Design review of the part built by this model. Coordinates are the model's own, in mm. A direction names the side the tool comes from. Coordinates: 2 decimals unless noted, no trailing zeros. Loops run counter-clockwise (first coordinate to the right, second up) from the corner with the lowest first, then second, coordinate; pieces in that order, holes last. Notation, with made-up numbers: M 12,57.5 L 27,57.5 A32 cw 27,84.5 Z; hole C 26,4 d11. An arc over 180 degrees is marked long. One line per item, written item: value.
```python
from build123d import *
from build123d.topology import SkipClean

# Parameters (mm, degrees)
SKETCH2_R                                = 10
SKETCH2_R_2                              = 6
SKETCH2_R_3                              = 5
BOSS_EXTRUDE1_DEPTH                      = 2
BOSS_EXTRUDE2_START                      = -3
SKETCH2_3_R                              = 21
SKETCH2_3_R_2                            = 20
SKETCH2_3_R_3                            = 17
SKETCH2_3_R_4                            = 10
SKETCH2_3_R_5                            = 6
SKETCH2_3_R_6                            = 5
BOSS_EXTRUDE2_DEPTH                      = 3
BOSS_EXTRUDE3_START                      = -4
SKETCH2_4_R                              = 6
SKETCH2_4_R_2                            = 5
BOSS_EXTRUDE3_DEPTH                      = 4
SKETCH2_6_R                              = 20
SKETCH2_6_R_2                            = 17
BOSS_EXTRUDE4_DEPTH                      = 14
CBORE_FOR_M12_HEX_HEAD_BOLT1_D           = 3.6
CBORE_FOR_M12_HEX_HEAD_BOLT1_CBORE_D     = 6.7
CBORE_FOR_M12_HEX_HEAD_BOLT1_CBORE_DEPTH = 1.65
CIRPATTERN1_COUNT                        = 3
RIB1_REACH                               = 44.5
SKETCH4_WALL_W                           = 101.866218182
SKETCH4_WALL_H                           = 2
CIRPATTERN2_COUNT                        = 6


with BuildPart() as part:
    # Sketch2 → Boss-Extrude1 (new body)
    # profile 1 of 2: a face of its own
    with BuildSketch(Plane(origin=(0, 0, 0), x_dir=(1, 0, 0), z_dir=(0, 1, 0))):
        with Locations(Location((0, 0, 0), (0, 0, 270))):
            Circle(SKETCH2_R)
        Circle(SKETCH2_R_2, mode=Mode.SUBTRACT)
    # profile 2 of 2: a face of its own
    with BuildSketch(Plane(origin=(0, 0, 0), x_dir=(1, 0, 0), z_dir=(0, 1, 0))):
        Circle(SKETCH2_R_2)
        with Locations(Location((0, 0, 0), (0, 0, 270))):
            Circle(SKETCH2_R_3, mode=Mode.SUBTRACT)
    extrude(amount=BOSS_EXTRUDE1_DEPTH)

    # Sketch2_3 → Boss-Extrude2 (add)
    # profile 1 of 8: a face of its own
    with BuildSketch(Plane(origin=(0, 0, 0), x_dir=(1, 0, 0), z_dir=(0, 1, 0)).offset(BOSS_EXTRUDE2_START)):
        with BuildLine():
            ThreePointArc((-15.163521733, -14.528166046), (-18.186533479, -10.5), (-20.163521733, -5.867912008))
            Line((-20.163521733, -5.867912008), (-24.150635095, -8.169872981))
            ThreePointArc((-24.150635095, -8.169872981), (-25.980762114, -15), (-19.150635095, -16.830127019))
            Line((-19.150635095, -16.830127019), (-15.163521733, -14.528166046))
        make_face()
    # profile 2 of 8: a face of its own
    with BuildSketch(Plane(origin=(0, 0, 0), x_dir=(1, 0, 0), z_dir=(0, 1, 0)).offset(BOSS_EXTRUDE2_START)):
        with BuildLine():
            Line((24.150635095, -8.169872981), (20.163521733, -5.867912008))
            ThreePointArc((20.163521733, -5.867912008), (18.186533479, -10.5), (15.163521733, -14.528166046))
            Line((15.163521733, -14.528166046), (19.150635095, -16.830127019))
            ThreePointArc((19.150635095, -16.830127019), (25.980762114, -15), (24.150635095, -8.169872981))
        make_face()
    # profile 3 of 8: a face of its own
    with BuildSketch(Plane(origin=(0, 0, 0), x_dir=(1, 0, 0), z_dir=(0, 1, 0)).offset(BOSS_EXTRUDE2_START)):
        with BuildLine():
            Line((5, 20.396078054), (5, 25))
            ThreePointArc((5, 25), (0, 30), (-5, 25))
            Line((-5, 25), (-5, 20.396078054))
            ThreePointArc((-5, 20.396078054), (0, 21), (5, 20.396078054))
        make_face()
    # profile 4 of 8: a face of its own
    with BuildSketch(Plane(origin=(0, 0, 0), x_dir=(1, 0, 0), z_dir=(0, 1, 0)).offset(BOSS_EXTRUDE2_START)):
        Circle(SKETCH2_3_R)
        Circle(SKETCH2_3_R_2, mode=Mode.SUBTRACT)
    # profile 5 of 8: a face of its own
    with BuildSketch(Plane(origin=(0, 0, 0), x_dir=(1, 0, 0), z_dir=(0, 1, 0)).offset(BOSS_EXTRUDE2_START)):
        Circle(SKETCH2_3_R_2)
        Circle(SKETCH2_3_R_3, mode=Mode.SUBTRACT)
    # profile 6 of 8: a face of its own
    with BuildSketch(Plane(origin=(0, 0, 0), x_dir=(1, 0, 0), z_dir=(0, 1, 0)).offset(BOSS_EXTRUDE2_START)):
        Circle(SKETCH2_3_R_3)
        with Locations(Location((0, 0, 0), (0, 0, 270))):
            Circle(SKETCH2_3_R_4, mode=Mode.SUBTRACT)
    # profile 7 of 8: a face of its own
    with BuildSketch(Plane(origin=(0, 0, 0), x_dir=(1, 0, 0), z_dir=(0, 1, 0)).offset(BOSS_EXTRUDE2_START)):
        with Locations(Location((0, 0, 0), (0, 0, 270))):
            Circle(SKETCH2_3_R_4)
        Circle(SKETCH2_3_R_5, mode=Mode.SUBTRACT)
    # profile 8 of 8: a face of its own
    with BuildSketch(Plane(origin=(0, 0, 0), x_dir=(1, 0, 0), z_dir=(0, 1, 0)).offset(BOSS_EXTRUDE2_START)):
        Circle(SKETCH2_3_R_5)
        with Locations(Location((0, 0, 0), (0, 0, 270))):
            Circle(SKETCH2_3_R_6, mode=Mode.SUBTRACT)
    extrude(amount=BOSS_EXTRUDE2_DEPTH)

    # Sketch2_4 → Boss-Extrude3 (add)
    with BuildSketch(Plane(origin=(0, 0, 0), x_dir=(1, 0, 0), z_dir=(0, 1, 0)).offset(BOSS_EXTRUDE3_START)):
        with Locations(Location((0, 0, 0), (0, 0, 270))):
            Circle(SKETCH2_4_R)
        with Locations(Location((0, 0, 0), (0, 0, 270))):
            Circle(SKETCH2_4_R_2, mode=Mode.SUBTRACT)
    extrude(amount=BOSS_EXTRUDE3_DEPTH)

    # Sketch2_6 → Boss-Extrude4 (add)
    with BuildSketch(Plane(origin=(0, 0, 0), x_dir=(1, 0, 0), z_dir=(0, 1, 0))):
        with Locations(Location((0, 0, 0), (0, 0, 270))):
            Circle(SKETCH2_6_R)
        with Locations(Location((0, 0, 0), (0, 0, 270))):
            Circle(SKETCH2_6_R_2, mode=Mode.SUBTRACT)
    extrude(amount=-BOSS_EXTRUDE4_DEPTH)

    # CBORE for M12 Hex Head Bolt1 (through all)
    with Locations(Plane(origin=(0, 0, -25), x_dir=(0, 0, 1), z_dir=(0, 1, 0))):
        with Locations((0, 0)):
            cbore_for_m12_hex_head_bolt1 = CounterBoreHole(CBORE_FOR_M12_HEX_HEAD_BOLT1_D / 2, CBORE_FOR_M12_HEX_HEAD_BOLT1_CBORE_D / 2, CBORE_FOR_M12_HEX_HEAD_BOLT1_CBORE_DEPTH)

    # CirPattern1: CBORE for M12 Hex Head Bolt1 ×3 about axis
    cirpattern1_axis = Axis((0, 0, 0), (0, 1, 0))
    for i in range(1, CIRPATTERN1_COUNT):
        add(cbore_for_m12_hex_head_bolt1.rotate(cirpattern1_axis, i * 360 / CIRPATTERN1_COUNT), mode=Mode.SUBTRACT)

    # Sketch4 wall → Rib1 (add, up to next)
    with BuildSketch(Plane(origin=(-11.5, -9, 0), x_dir=(0.739940073396, 0.672672793996, 0), z_dir=(-0.672672793996, 0.739940073396, 0)), mode=Mode.PRIVATE) as rib1_sk1:
        Rectangle(SKETCH4_WALL_W, SKETCH4_WALL_H)
    rib1_tool1 = extrude(rib1_sk1.sketch, amount=RIB1_REACH, mode=Mode.PRIVATE) - part.part
    rib1 = rib1_tool1.solids().sort_by_distance((-11.5, -9, 0))[0]
    add(rib1)

    # CirPattern2: Rib1 ×6 about axis
    with SkipClean():  # the faces are left unmerged after this step: merging them gives an invalid solid
        cirpattern2_axis = Axis((0, 0, 0), (0, 1, 0))
        for i in range(1, CIRPATTERN2_COUNT):
            add(rib1.rotate(cirpattern2_axis, i * 360 / CIRPATTERN2_COUNT))


solid = part.part
```
(1) To check wall thickness, follow line 1 along X through (y, z) = (-0.75, 12.5); line 2 along X through (y, z) = (-0.4, -25); line 3 along Z through (x, y) = (11.5, -6.5). State the ranges of each line that lie inside material, in increasing order. Write a range as [from, to].
Reply:
line 1: x = [-26.65, -25], [-18.3, 18.3], [25, 26.65]
line 2: x = [-5, -3.35], [3.35, 5]
line 3: z = [-16.36, -12.52], [-1, 1], [12.52, 16.36]
(2) We need section D-D on z = 12.5. State how many separate pieces and enclosed holes the cut face has, then the cut area to 3 significant figures.
Reply:
separate pieces: 3
enclosed holes: 0
area: 258 mm2
(3) We need section A-A on y = -10.5. State the section outline as (x, z) points, then the cut area to 3 significant figures.
Reply:
outline: C 0,0 d40; hole M -16.97,-1 A17 ccw -9.35,-14.2 L -7.44,-10.89 L -5.71,-11.89 L -7.62,-15.2 A17 ccw 7.62,-15.2 L 5.71,-11.89 L 7.44,-10.89 L 9.35,-14.2 A17 ccw 16.97,-1 L 13.15,-1 L 13.15,1 L 16.97,1 A17 ccw 9.35,14.2 L 7.44,10.89 L 5.71,11.89 L 7.62,15.2 A17 ccw -7.62,15.2 L -5.71,11.89 L -7.44,10.89 L -9.35,14.2 A17 ccw -16.97,1 L -13.15,1 L -13.15,-1 Z
area: 395 mm2
(4) Tool access review of faces 3 (the flat face through (22.185, -1.521, 7.035)), 4 (the flat face through (21.1, -1.65, 10.5)), 5 (the flat face through (5.824, -6.518, 12.087)), 6 (the cylindrical face through (-18.07, -1.52, -10.7)), 7 (the flat face through (-17.185, -1.521, 15.695)): name each direction out of +Z, -Z, +X, -X, +Y, -Y from which nothing blocks a thin tool from reaching the whole face with its end or side.
Reply:
face 3: +X, +Y, -Y
face 4: +Y
face 5: -Y
face 6: -X, +Y, -Y
face 7: +Z, +Y, -Y
(5) Insertion check: pin 1 (8 mm diameter, centred on x = 20.5, y = -7, fed in from -Z); pin 2 (1.5 mm diameter, centred on y = -9, z = 12, fed in from -X); pin 3 (5 mm diameter, centred on y = -6.5, z = 6.5, fed in from -X). Each pin has a flat end and moves straight along its axis. Give the tip position at first contact, or say it passes through.
Reply:
pin 1: stops at z = -11.3
pin 2: stops at x = -16.54
pin 3: stops at x = -19.6
(6) Mouldability with a two-part tool opening along Z and no side actions: class faces 1 (the cylindrical face through (-22.746, -2.334, 13.928)), 2 (the flat face through (17.129, -1.521, 15.663)) as released by +Z, released by -Z, zero draft, split by the parting line, or undercut.
Reply:
face 1: undercut
face 2: released by +Z
(7) We need section B-B on x = -12. State the section outline as (y, z) points, then the cut area to 3 significant figures.
Reply:
outline: M -14,-16 L -3,-16 L -3,-17.23 L 0,-17.23 L 0,17.23 L -3,17.23 L -3,16 L -14,16 L -14,12.04 L -3,12.04 L -3,1 L -9.45,1 L -9.45,-1 L -3,-1 L -3,-12.04 L -14,-12.04 Z
area: 203 mm2
(8) We need section C-C on z = -11.5. State the section outline as (x, y) points, then the cut area to 3 significant figures.
Reply:
outline: M -17.57,-3 L -16.36,-3 L -16.36,-14 L -12.52,-14 L -12.52,-3 L -7.79,-3 L -7.79,-11.14 L -5.48,-10.09 L -5.48,-3 L 5.48,-3 L 5.48,-10.09 L 7.79,-11.14 L 7.79,-3 L 12.52,-3 L 12.52,-14 L 16.36,-14 L 16.36,-3 L 17.57,-3 L 17.57,0 L -17.57,0 Z
area: 225 mm2
